Work out the finished part from the listing and answer in its coordinate system (mm). A direction names the side the tool comes from. Give positions to 0.01 mm unless a question says otherwise; leave off trailing zeros. Loops run counter-clockwise (first coordinate to the right, second up) from the corner with the lowest first, then second, coordinate; pieces in that order, holes last. Notation, with made-up numbers: M 10,64.5 L 26,64.5 A8 ccw 26,75.5 Z; hole C 42,-13 d1. An arc over 180 degrees is marked long. Answer in a Markdown table with one row per item. Add a question column.
from build123d import *

# Parameters (mm, degrees)
BOSS_EXTRUDE1_DEPTH     = 6.5
SKETCH2_R               = 7
BOSS_EXTRUDE2_DEPTH     = 10
SKETCH3_R               = 5.5
CUT_EXTRUDE1_DEPTH      = 3
SKETCH4_R               = 2.25
CUT_EXTRUDE2_DEPTH      = 1
CUT_EXTRUDE2_DEPTH_BACK = 17.5
FILLET1_R               = 3


with BuildPart() as part:
    # Sketch1 → Boss-Extrude1 (new body)
    with BuildSketch(Plane(origin=(0, 0, 0), x_dir=(0, 0, -1), z_dir=(1, 0, 0))):
        with BuildLine():
            Line((1.815874997, 47.835924448), (8.381939498, 53.345506749))
            ThreePointArc((8.381939498, 53.345506749), (13.976228436, 52.15999462), (19.413780836, 50.389533771))
            Line((19.413780836, 50.389533771), (22.345368346, 42.335063284))
            ThreePointArc((22.345368346, 42.335063284), (23.5875, 40.854748424), (25.490556102, 40.519188287))
            Line((25.490556102, 40.519188287), (33.931725912, 42.007594273))
            ThreePointArc((33.931725912, 42.007594273), (38.183766184, 38.183766184), (42.007594273, 33.931725912))
            Line((42.007594273, 33.931725912), (40.519188287, 25.490556102))
            ThreePointArc((40.519188287, 25.490556102), (40.854748424, 23.5875), (42.335063284, 22.345368346))
            Line((42.335063284, 22.345368346), (50.389533771, 19.413780836))
            ThreePointArc((50.389533771, 19.413780836), (52.15999462, 13.976228436), (53.345506749, 8.381939498))
            Line((53.345506749, 8.381939498), (47.835924448, 1.815874997))
            ThreePointArc((47.835924448, 1.815874997), (47.175, 0), (47.835924448, -1.815874997))
            Line((47.835924448, -1.815874997), (53.345506749, -8.381939498))
            ThreePointArc((53.345506749, -8.381939498), (52.15999462, -13.976228436), (50.389533771, -19.413780836))
            Line((50.389533771, -19.413780836), (42.335063284, -22.345368346))
            ThreePointArc((42.335063284, -22.345368346), (40.854748424, -23.5875), (40.519188287, -25.490556102))
            Line((40.519188287, -25.490556102), (42.007594273, -33.931725912))
            ThreePointArc((42.007594273, -33.931725912), (38.183766184, -38.183766184), (33.931725912, -42.007594273))
            Line((33.931725912, -42.007594273), (25.490556102, -40.519188287))
            ThreePointArc((25.490556102, -40.519188287), (23.5875, -40.854748424), (22.345368346, -42.335063284))
            Line((22.345368346, -42.335063284), (19.413780836, -50.389533771))
            ThreePointArc((19.413780836, -50.389533771), (13.976228436, -52.15999462), (8.381939498, -53.345506749))
            Line((8.381939498, -53.345506749), (1.815874997, -47.835924448))
            ThreePointArc((1.815874997, -47.835924448), (0, -47.175), (-1.815874997, -47.835924448))
            Line((-1.815874997, -47.835924448), (-8.381939498, -53.345506749))
            ThreePointArc((-8.381939498, -53.345506749), (-13.976228436, -52.15999462), (-19.413780836, -50.389533771))
            Line((-19.413780836, -50.389533771), (-22.345368346, -42.335063284))
            ThreePointArc((-22.345368346, -42.335063284), (-23.5875, -40.854748424), (-25.490556102, -40.519188287))
            Line((-25.490556102, -40.519188287), (-33.931725912, -42.007594273))
            ThreePointArc((-33.931725912, -42.007594273), (-38.183766184, -38.183766184), (-42.007594273, -33.931725912))
            Line((-42.007594273, -33.931725912), (-40.519188287, -25.490556102))
            ThreePointArc((-40.519188287, -25.490556102), (-40.854748424, -23.5875), (-42.335063284, -22.345368346))
            Line((-42.335063284, -22.345368346), (-50.389533771, -19.413780836))
            ThreePointArc((-50.389533771, -19.413780836), (-52.15999462, -13.976228436), (-53.345506749, -8.381939498))
            Line((-53.345506749, -8.381939498), (-47.835924448, -1.815874997))
            ThreePointArc((-47.835924448, -1.815874997), (-47.175, 0), (-47.835924448, 1.815874997))
            Line((-47.835924448, 1.815874997), (-53.345506749, 8.381939498))
            ThreePointArc((-53.345506749, 8.381939498), (-52.15999462, 13.976228436), (-50.389533771, 19.413780836))
            Line((-50.389533771, 19.413780836), (-42.335063284, 22.345368346))
            ThreePointArc((-42.335063284, 22.345368346), (-40.854748424, 23.5875), (-40.519188287, 25.490556102))
            Line((-40.519188287, 25.490556102), (-42.007594273, 33.931725912))
            ThreePointArc((-42.007594273, 33.931725912), (-38.183766184, 38.183766184), (-33.931725912, 42.007594273))
            Line((-33.931725912, 42.007594273), (-25.490556102, 40.519188287))
            ThreePointArc((-25.490556102, 40.519188287), (-23.5875, 40.854748424), (-22.345368346, 42.335063284))
            Line((-22.345368346, 42.335063284), (-19.413780836, 50.389533771))
            ThreePointArc((-19.413780836, 50.389533771), (-13.976228436, 52.15999462), (-8.381939498, 53.345506749))
            Line((-8.381939498, 53.345506749), (-1.815874997, 47.835924448))
            ThreePointArc((-1.815874997, 47.835924448), (0, 47.175), (1.815874997, 47.835924448))
        make_face()
    extrude(amount=BOSS_EXTRUDE1_DEPTH)

    # Sketch2 → Boss-Extrude2 (add)
    with BuildSketch(Plane(origin=(6.5, 0, 0), x_dir=(0, 0, -1), z_dir=(1, 0, 0))):
        Circle(SKETCH2_R)
    extrude(amount=BOSS_EXTRUDE2_DEPTH)

    # Sketch3 → Cut-Extrude1 (cut)
    with BuildSketch(Plane(origin=(16.5, 0, 0), x_dir=(0, 0, -1), z_dir=(1, 0, 0))):
        Circle(SKETCH3_R)
    extrude(amount=-CUT_EXTRUDE1_DEPTH, mode=Mode.SUBTRACT)

    # Sketch4 → Cut-Extrude2 (cut, two sides)
    with BuildSketch(Plane.ZY) as cut_extrude2_sk:
        Circle(SKETCH4_R)
    extrude(amount=CUT_EXTRUDE2_DEPTH, mode=Mode.SUBTRACT)
    extrude(cut_extrude2_sk.sketch, amount=-CUT_EXTRUDE2_DEPTH_BACK, mode=Mode.SUBTRACT)

    # Fillet1
    fillet1_edges = [part.edges().sort_by_distance(p)[0] for p in [
        (6.5, -52.15999462, 13.976228436),
        (6.5, -52.15999462, -13.976228436),
        (6.5, 52.15999462, -13.976228436),
        (6.5, -38.183766184, -38.183766184),
        (6.5, -13.976228436, -52.15999462),
        (6.5, 13.976228436, -52.15999462),
        (6.5, 38.183766184, -38.183766184),
        (6.5, 52.15999462, 13.976228436),
        (6.5, 38.183766184, 38.183766184),
        (6.5, 13.976228436, 52.15999462),
        (6.5, -13.976228436, 52.15999462),
        (6.5, -38.183766184, 38.183766184),
    ]]
    fillet(fillet1_edges, radius=FILLET1_R)


solid = part.part
(1) Section D-D, the plane y = -44.5 is taken. Determine the outline of the cut face in (x, z).
(2) Section C-C, the plane x = 11.5 is taken. Determine the outline of the cut face in (y, z).
(3) Each of these flat-tipped pins is pushed along its axis until it touches: P1, Ø4, axis at y = 10, z = 21.5, coming from the +X side; P2, Ø17.5, axis at y = 0, z = 0, coming from the +X side; P3, Ø2, axis at x = 6.5, z = -20.5, coming from the +Y side; P4, Ø1, axis at x = 5, z = 12, coming from the +Y side. Where does it stop, or does it pass through?
(4) The mould has two halves that part along Z. Classify faces 1 (the face through (3.2, -46.42, 20.86)), 2 (the face through (3.204, 0.028, -47.175)), 3 (the face through (3.2, 40.84, 23.61)): pulls with the +Z half, pulls with the -Z half, needs draft (parallel to the pull), parting line crosses it, or undercut.
(5) Which of the six approach directions +Z, -Z, +X, -X, +Y, -Y give full straight-line access (tool end or side, diameter ignored) to faces 4 (the face through (3.204, 29.652, 41.253)), 5 (the face through (11.43, -2.681, -6.466)), 6 (the face through (3.2, -50.55, 5.05)), 7 (the face through (3.204, -29.652, -41.253))?
(6) Consider line 1 along Y through (x, z) = (9, 0); line 2 along Y through (x, z) = (4.5, 0) (3 decimals); line 3 along X through (y, z) = (-10, 1). Determine where each line is inside the solid, lowest interval first. Write a range as from..to.
(7) Section A-A, the plane y = 0 is taken. Determine the outline of the cut face in (x, z) (3 decimals), and give its area (3 significant figures).
Numbers:
| question | item | result |
|---|---|---|
| 1 | outline | M 0,-21.56 L 6.5,-21.56 L 6.5,21.56 L 0,21.56 Z |
| 2 | outline | C 0,0 d14; hole C 0,0 d4.5 |
| 3 | P1 | stops at x = 6.5 |
| 3 | P2 | stops at x = 16.5 |
| 3 | P3 | stops at y = 49.15 |
| 3 | P4 | stops at y = 52.51 |
| 4 | face 1 | pulls with the +Z half |
| 4 | face 2 | pulls with the -Z half |
| 4 | face 3 | undercut |
| 5 | face 4 | +Z, +X, -X |
| 5 | face 5 | +X |
| 5 | face 6 | +X, -X, -Y |
| 5 | face 7 | -Z, +X, -X |
| 6 | line 1 | y = -7..-2.25, 2.25..7 |
| 6 | line 2 | y = -47.175..-2.25, 2.25..47.175 |
| 6 | line 3 | x = 0..6.5 |
| 7 | outline | M 0,-47.175 L 6.5,-47.175 L 6.5,-7 L 16.5,-7 L 16.5,-5.5 L 13.5,-5.5 L 13.5,-2.25 L 0,-2.25 Z; M 0,2.25 L 13.5,2.25 L 13.5,5.5 L 16.5,5.5 L 16.5,7 L 6.5,7 L 6.5,47.175 L 0,47.175 Z |
| 7 | area | 660 mm² |
